The listing builds one solid part. Answer for the finished solid, in the listing's coordinates (mm). Coordinates: 2 decimals unless noted, no trailing zeros. Return JSON: item names as keys, results as strings.
from build123d import *

# Parameters (mm, degrees)
SKETCH_1_W          = 919.725090766
SKETCH_1_H          = 80
EXTRUDE_1_DEPTH     = 3
CUT_EXTRUDE_1_DEPTH = 3


with BuildPart() as part:
    # Эскиз1 → Бобышка-Вытянуть1 (new body)
    with BuildSketch(Plane.XY):
        with Locations((-419.862545383, 0)):
            Rectangle(SKETCH_1_W, SKETCH_1_H)
        with BuildLine():
            Line((-815.471010416, -25), (-864.528989584, -25))
            ThreePointArc((-864.528989584, -25), (-864.148088497, -25.716125252), (-864.016504294, -26.516504295))
            ThreePointArc((-864.016504294, -26.516504295), (-868.757180614, -27.625273717), (-865, -24.528989584))
            Line((-865, -24.528989584), (-865, 24.528989584))
            ThreePointArc((-865, 24.528989584), (-868.757180614, 27.625273717), (-864.016504295, 26.516504294))
            ThreePointArc((-864.016504295, 26.516504294), (-864.148088497, 25.716125252), (-864.528989584, 25))
            Line((-864.528989584, 25), (-815.471010416, 25))
            ThreePointArc((-815.471010416, 25), (-814.283874748, 28.884920092), (-810.983495706, 26.516504294))
            ThreePointArc((-810.983495706, 26.516504294), (-812.374726283, 24.275827975), (-815, 24.528989584))
            Line((-815, 24.528989584), (-815, -24.528989584))
            ThreePointArc((-815, -24.528989584), (-812.374726283, -24.275827975), (-810.983495705, -26.516504294))
            ThreePointArc((-810.983495705, -26.516504294), (-814.283874748, -28.884920092), (-815.471010416, -25))
        make_face(mode=Mode.SUBTRACT)
        with BuildLine():
            Line((-695.471010416, -25), (-744.528989584, -25))
            ThreePointArc((-744.528989584, -25), (-744.148088497, -25.716125252), (-744.016504294, -26.516504295))
            ThreePointArc((-744.016504294, -26.516504295), (-748.757180614, -27.625273717), (-745, -24.528989584))
            Line((-745, -24.528989584), (-745, 24.528989584))
            ThreePointArc((-745, 24.528989584), (-748.757180614, 27.625273717), (-744.016504295, 26.516504294))
            ThreePointArc((-744.016504295, 26.516504294), (-744.148088497, 25.716125252), (-744.528989584, 25))
            Line((-744.528989584, 25), (-695.471010416, 25))
            ThreePointArc((-695.471010416, 25), (-694.283874748, 28.884920092), (-690.983495706, 26.516504295))
            ThreePointArc((-690.983495706, 26.516504295), (-692.374726283, 24.275827975), (-695, 24.528989584))
            Line((-695, 24.528989584), (-695, -24.528989584))
            ThreePointArc((-695, -24.528989584), (-692.374726283, -24.275827975), (-690.983495705, -26.516504294))
            ThreePointArc((-690.983495705, -26.516504294), (-694.283874748, -28.884920092), (-695.471010416, -25))
        make_face(mode=Mode.SUBTRACT)
        with BuildLine():
            Line((-575.471010416, -25), (-624.528989584, -25))
            ThreePointArc((-624.528989584, -25), (-624.148088497, -25.716125252), (-624.016504294, -26.516504295))
            ThreePointArc((-624.016504294, -26.516504295), (-628.757180614, -27.625273717), (-625, -24.528989584))
            Line((-625, -24.528989584), (-625, 24.528989584))
            ThreePointArc((-625, 24.528989584), (-628.757180614, 27.625273717), (-624.016504295, 26.516504294))
            ThreePointArc((-624.016504295, 26.516504294), (-624.148088497, 25.716125252), (-624.528989584, 25))
            Line((-624.528989584, 25), (-575.471010416, 25))
            ThreePointArc((-575.471010416, 25), (-574.283874748, 28.884920092), (-570.983495706, 26.516504295))
            ThreePointArc((-570.983495706, 26.516504295), (-572.374726283, 24.275827975), (-575, 24.528989584))
            Line((-575, 24.528989584), (-575, -24.528989584))
            ThreePointArc((-575, -24.528989584), (-572.374726283, -24.275827975), (-570.983495705, -26.516504294))
            ThreePointArc((-570.983495705, -26.516504294), (-574.283874748, -28.884920092), (-575.471010416, -25))
        make_face(mode=Mode.SUBTRACT)
        with BuildLine():
            Line((-455.471010416, -25), (-504.528989584, -25))
            ThreePointArc((-504.528989584, -25), (-504.148088497, -25.716125252), (-504.016504294, -26.516504295))
            ThreePointArc((-504.016504294, -26.516504295), (-508.757180614, -27.625273717), (-505, -24.528989584))
            Line((-505, -24.528989584), (-505, 24.528989584))
            ThreePointArc((-505, 24.528989584), (-508.757180614, 27.625273717), (-504.016504295, 26.516504294))
            ThreePointArc((-504.016504295, 26.516504294), (-504.148088497, 25.716125252), (-504.528989584, 25))
            Line((-504.528989584, 25), (-455.471010416, 25))
            ThreePointArc((-455.471010416, 25), (-454.283874748, 28.884920092), (-450.983495706, 26.516504295))
            ThreePointArc((-450.983495706, 26.516504295), (-452.374726283, 24.275827975), (-455, 24.528989584))
            Line((-455, 24.528989584), (-455, -24.528989584))
            ThreePointArc((-455, -24.528989584), (-452.374726283, -24.275827975), (-450.983495705, -26.516504294))
            ThreePointArc((-450.983495705, -26.516504294), (-454.283874748, -28.884920092), (-455.471010416, -25))
        make_face(mode=Mode.SUBTRACT)
        with BuildLine():
            Line((-335.471010416, -25), (-384.528989584, -25))
            ThreePointArc((-384.528989584, -25), (-384.148088497, -25.716125252), (-384.016504294, -26.516504295))
            ThreePointArc((-384.016504294, -26.516504295), (-388.757180614, -27.625273717), (-385, -24.528989584))
            Line((-385, -24.528989584), (-385, 24.528989584))
            ThreePointArc((-385, 24.528989584), (-388.757180614, 27.625273717), (-384.016504295, 26.516504294))
            ThreePointArc((-384.016504295, 26.516504294), (-384.148088497, 25.716125252), (-384.528989584, 25))
            Line((-384.528989584, 25), (-335.471010416, 25))
            ThreePointArc((-335.471010416, 25), (-334.283874748, 28.884920092), (-330.983495706, 26.516504295))
            ThreePointArc((-330.983495706, 26.516504295), (-332.374726283, 24.275827975), (-335, 24.528989584))
            Line((-335, 24.528989584), (-335, -24.528989584))
            ThreePointArc((-335, -24.528989584), (-332.374726283, -24.275827975), (-330.983495705, -26.516504294))
            ThreePointArc((-330.983495705, -26.516504294), (-334.283874748, -28.884920092), (-335.471010416, -25))
        make_face(mode=Mode.SUBTRACT)
        with BuildLine():
            Line((-215.471010416, -25), (-264.528989584, -25))
            ThreePointArc((-264.528989584, -25), (-264.148088497, -25.716125252), (-264.016504294, -26.516504295))
            ThreePointArc((-264.016504294, -26.516504295), (-268.757180614, -27.625273717), (-265, -24.528989584))
            Line((-265, -24.528989584), (-265, 24.528989584))
            ThreePointArc((-265, 24.528989584), (-268.757180614, 27.625273717), (-264.016504295, 26.516504294))
            ThreePointArc((-264.016504295, 26.516504294), (-264.148088497, 25.716125252), (-264.528989584, 25))
            Line((-264.528989584, 25), (-215.471010416, 25))
            ThreePointArc((-215.471010416, 25), (-214.283874748, 28.884920092), (-210.983495706, 26.516504295))
            ThreePointArc((-210.983495706, 26.516504295), (-212.374726283, 24.275827975), (-215, 24.528989584))
            Line((-215, 24.528989584), (-215, -24.528989584))
            ThreePointArc((-215, -24.528989584), (-212.374726283, -24.275827975), (-210.983495705, -26.516504294))
            ThreePointArc((-210.983495705, -26.516504294), (-214.283874748, -28.884920092), (-215.471010416, -25))
        make_face(mode=Mode.SUBTRACT)
        with BuildLine():
            Line((-95.471010416, -25), (-144.528989584, -25))
            ThreePointArc((-144.528989584, -25), (-144.148088497, -25.716125252), (-144.016504294, -26.516504295))
            ThreePointArc((-144.016504294, -26.516504295), (-148.757180614, -27.625273717), (-145, -24.528989584))
            Line((-145, -24.528989584), (-145, 24.528989584))
            ThreePointArc((-145, 24.528989584), (-148.757180614, 27.625273717), (-144.016504295, 26.516504294))
            ThreePointArc((-144.016504295, 26.516504294), (-144.148088497, 25.716125252), (-144.528989584, 25))
            Line((-144.528989584, 25), (-95.471010416, 25))
            ThreePointArc((-95.471010416, 25), (-94.283874748, 28.884920092), (-90.983495706, 26.516504295))
            ThreePointArc((-90.983495706, 26.516504295), (-92.374726283, 24.275827975), (-95, 24.528989584))
            Line((-95, 24.528989584), (-95, -24.528989584))
            ThreePointArc((-95, -24.528989584), (-92.374726283, -24.275827975), (-90.983495705, -26.516504294))
            ThreePointArc((-90.983495705, -26.516504294), (-94.283874748, -28.884920092), (-95.471010416, -25))
        make_face(mode=Mode.SUBTRACT)
        with BuildLine():
            Line((24.528989584, -25), (-24.528989584, -25))
            ThreePointArc((-24.528989584, -25), (-24.148088497, -25.716125252), (-24.016504294, -26.516504295))
            ThreePointArc((-24.016504294, -26.516504295), (-28.757180614, -27.625273717), (-25, -24.528989584))
            Line((-25, -24.528989584), (-25, 24.528989584))
            ThreePointArc((-25, 24.528989584), (-28.757180614, 27.625273717), (-24.016504295, 26.516504294))
            ThreePointArc((-24.016504295, 26.516504294), (-24.148088497, 25.716125252), (-24.528989584, 25))
            Line((-24.528989584, 25), (24.528989584, 25))
            ThreePointArc((24.528989584, 25), (25.716125252, 28.884920092), (29.016504294, 26.516504295))
            ThreePointArc((29.016504294, 26.516504295), (27.625273717, 24.275827975), (25, 24.528989584))
            Line((25, 24.528989584), (25, -24.528989584))
            ThreePointArc((25, -24.528989584), (27.625273717, -24.275827975), (29.016504295, -26.516504294))
            ThreePointArc((29.016504295, -26.516504294), (25.716125252, -28.884920092), (24.528989584, -25))
        make_face(mode=Mode.SUBTRACT)
    extrude(amount=EXTRUDE_1_DEPTH)

    # Эскиз2 → Вырез-Вытянуть1 (cut)
    with BuildSketch(Plane(origin=(0, 0, 0), x_dir=(-1, 0, 0), z_dir=(0, 0, -1))):
        with BuildLine():
            Line((62, 20), (62, -20))
            ThreePointArc((62, -20), (60, -22), (58, -20))
            Line((58, -20), (58, 20))
            ThreePointArc((58, 20), (60, 22), (62, 20))
        make_face()
        with BuildLine():
            Line((182, 20), (182, -20))
            ThreePointArc((182, -20), (180, -22), (178, -20))
            Line((178, -20), (178, 20))
            ThreePointArc((178, 20), (180, 22), (182, 20))
        make_face()
        with BuildLine():
            Line((302, 20), (302, -20))
            ThreePointArc((302, -20), (300, -22), (298, -20))
            Line((298, -20), (298, 20))
            ThreePointArc((298, 20), (300, 22), (302, 20))
        make_face()
        with BuildLine():
            Line((422, 20), (422, -20))
            ThreePointArc((422, -20), (420, -22), (418, -20))
            Line((418, -20), (418, 20))
            ThreePointArc((418, 20), (420, 22), (422, 20))
        make_face()
        with BuildLine():
            Line((542, 20), (542, -20))
            ThreePointArc((542, -20), (540, -22), (538, -20))
            Line((538, -20), (538, 20))
            ThreePointArc((538, 20), (540, 22), (542, 20))
        make_face()
        with BuildLine():
            Line((662, 20), (662, -20))
            ThreePointArc((662, -20), (660, -22), (658, -20))
            Line((658, -20), (658, 20))
            ThreePointArc((658, 20), (660, 22), (662, 20))
        make_face()
        with BuildLine():
            Line((782, 20), (782, -20))
            ThreePointArc((782, -20), (780, -22), (778, -20))
            Line((778, -20), (778, 20))
            ThreePointArc((778, 20), (780, 22), (782, 20))
        make_face()
    extrude(amount=-CUT_EXTRUDE_1_DEPTH, mode=Mode.SUBTRACT)


solid = part.part
1. The part is cut by section A-A on z = 1.2. Give the number of separate pieces and of enclosed holes in the cut face, and give its area (3 significant figures).
Answer block:
{"separate pieces": "1", "enclosed holes": "15", "area": "51,700 mm2"}
2. Consider line 1 (Y direction, x = -213.5, z = 2.1); line 2 (Y direction, x = -236, z = 2.6); line 3 (Y direction, x = -28.5, z = 2.35). Determine where each line is inside the solid, lowest interval first. Write a range as from..to.
Answer block:
{"line 1": "y = -40..-29.02, -24.02..24.02, 29.02..40", "line 2": "y = -40..-25, 25..40", "line 3": "y = -40..-28.04, -24.99..24.99, 28.04..40"}
3. This flat-tipped pin is pushed along its axis until it touches: pin 1 Ø4.5 at (x, y) = (-453.48, -26.52) entering from +Z. Where does it stop, or does it pass through?
Answer block:
{"pin 1": "passes through"}
